Design review of the part built by this model. Coordinates are the model's own, in mm. Face numbers are marked on the shaded views. Give positions to 0.01 mm unless a question says otherwise; leave off trailing zeros. Write each loop counter-clockwise with the first axis right and the second up, starting at its lowest first coordinate (ties: lowest second). Pieces come first, ordered by that corner, then holes. Notation, with made-up numbers: (12, 81) -> (55, 81) arc R25 ccw to (55, 120) -> close; hole circle Ø9 at (39.25, 75.25). An arc over 180 degrees is marked (long way). Write each question's results on one line, items separated by ' | '. Start each with the question number.
(1) Take a section at A-A (y = 12). State the section outline as (x, z) points, plus the area to 3 significant figures.
(2) Mouldability with a two-part tool opening along Z and no side actions: class the marked faces 1 and 2 as released by +Z, released by -Z, zero draft, split by the parting line, or undercut.
(3) Clearance check with flat-ended pins moving along their axes: pin 1 (2 mm diameter, centred on y = 34, z = -10, fed in from -X); pin 2 (1.5 mm diameter, centred on y = 63, z = -4, fed in from -X); pin 3 (1 mm diameter, centred on y = 137.5, z = 11, fed in from +X). State where each tip first meets the part, or that it passes through.
(4) Take a section at B-B (y = 123.5). State the section outline as (x, z) points, plus the area to 3 significant figures.
(5) To check wall thickness, follow probe 1 along Z at (x, y) = (0, 84); probe 2 along Z at (x, y) = (0, 93.5); probe 3 along X at (y, z) = (89, 3). State the ranges of each line that lie inside material, in increasing order.
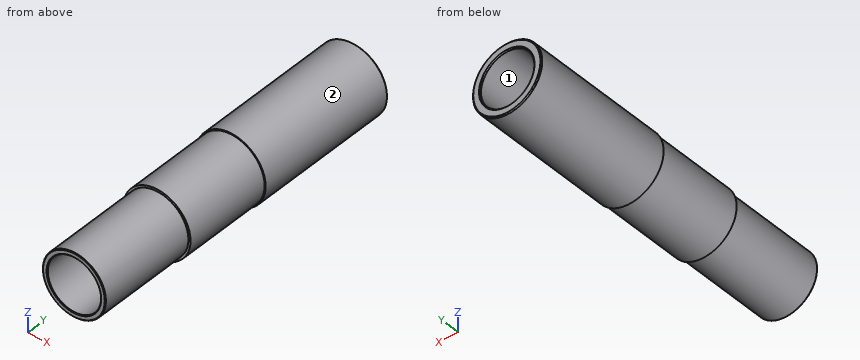
from build123d import *

# Parameters (mm, degrees)
SKETCH1_R           = 16
SKETCH1_R_2         = 12.7
BOSS_EXTRUDE1_DEPTH = 160
CHAMFER2_SIZE       = 0.3
SKETCH3_R           = 17.5
SKETCH3_R_2         = 15
CUT_EXTRUDE2_DEPTH  = 47.56
CHAMFER3_SIZE       = 0.3
SKETCH2_R           = 16.5
SKETCH2_R_2         = 12.7
BOSS_EXTRUDE3_DEPTH = 70
CHAMFER4_SIZE       = 0.5


with BuildPart() as part:
    # Sketch1 → Boss-Extrude1 (new body)
    with BuildSketch(Plane(origin=(0, 0, 0), x_dir=(1, 0, 0), z_dir=(0, 1, 0))):
        Circle(SKETCH1_R)
        Circle(SKETCH1_R_2, mode=Mode.SUBTRACT)
    extrude(amount=BOSS_EXTRUDE1_DEPTH)

    # Chamfer2
    chamfer2_edges = [part.edges().sort_by_distance(p)[0] for p in [
        (-12.7, 0, 0),
        (-12.7, 160, 0),
    ]]
    chamfer(chamfer2_edges, length=CHAMFER2_SIZE)

    # Sketch3 → Cut-Extrude2 (cut)
    with BuildSketch(Plane.XZ):
        Circle(SKETCH3_R)
        Circle(SKETCH3_R_2, mode=Mode.SUBTRACT)
    extrude(amount=-CUT_EXTRUDE2_DEPTH, mode=Mode.SUBTRACT)

    # Chamfer3
    chamfer3_edges = [part.edges().sort_by_distance(p)[0] for p in [
        (-15, 0, 0),
    ]]
    chamfer(chamfer3_edges, length=CHAMFER3_SIZE)

    # Sketch2 → Boss-Extrude3 (add)
    with BuildSketch(Plane(origin=(0, 160, 0), x_dir=(1, 0, 0), z_dir=(0, 1, 0))):
        Circle(SKETCH2_R)
        Circle(SKETCH2_R_2, mode=Mode.SUBTRACT)
    extrude(amount=-BOSS_EXTRUDE3_DEPTH)

    # Chamfer4
    chamfer4_edges = [part.edges().sort_by_distance(p)[0] for p in [
        (-16.5, 160, 0),
        (-12.7, 160, 0),
    ]]
    chamfer(chamfer4_edges, length=CHAMFER4_SIZE)


solid = part.part
Report:
1) outline: circle Ø30 at (0, 0); hole circle Ø25.4 at (0, 0) | area: 200 mm2
2) face 1: undercut | face 2: split by the parting line
3) pin 1: x = -12 | pin 2: x = -15.67 | pin 3: x = 12.73
4) outline: circle Ø33 at (0, 0); hole circle Ø25.4 at (0, 0) | area: 349 mm2
5) probe 1: -16 to -12.7, 12.7 to 16 | probe 2: -16.5 to -12.7, 12.7 to 16.5 | probe 3: -15.72 to -12.34, 12.34 to 15.72
